```python
from build123d import *

# Parameters (mm, degrees)
SKETCH1_R                = 3.2639
BOSS_EXTRUDE1_DEPTH      = 6.35
SKETCH2_R                = 2.0193
CUT_EXTRUDE1_DEPTH       = 6.35
SKETCH3_R                = 2.0193
CUT_EXTRUDE2_DEPTH       = 6.35
SKETCH5_R                = 2.0193
CUT_EXTRUDE3_DEPTH       = 6.35
SKETCH6_R                = 14.2875
CUT_EXTRUDE4_DEPTH       = 7.35
SKETCH7_R                = 3.2639
CUT_EXTRUDE5_DEPTH       = 7.35
F_0_257_DIAMETER_HOLE1_D = 6.5278
FILLET1_R                = 3.175
FILLET2_R                = 3.175


with BuildPart() as part:
    # Sketch1 → Boss-Extrude1 (new body)
    with BuildSketch(Plane.XY):
        with BuildLine():
            Line((-12.7, 76.2), (12.7, 76.2))
            Line((12.7, 76.2), (12.7, -76.2))
            Line((12.7, -76.2), (3.175, -76.2))
            Line((3.175, -76.2), (-7.968733256, -102.786346034))
            ThreePointArc((-7.968733256, -102.786346034), (-15.132721636, -107.653920671), (-22.482997382, -103.072495258))
            Line((-22.482997382, -103.072495258), (-35.013847715, -76.2))
            Line((-35.013847715, -76.2), (-114.3, -76.2))
            Line((-114.3, -76.2), (-114.3, -25.4))
            Line((-114.3, -25.4), (-12.7, 76.2))
        make_face()
        with Locations((-15.289179323, -99.717962805)):
            Circle(SKETCH1_R, mode=Mode.SUBTRACT)
        with Locations((-20.656431247, -88.20785391)):
            Circle(SKETCH1_R, mode=Mode.SUBTRACT)
    extrude(amount=BOSS_EXTRUDE1_DEPTH)

    # Sketch2 → Cut-Extrude1 (cut)
    with BuildSketch(Plane.XY.offset(6.35)):
        with Locations((4.7625, 68.2625)):
            Circle(SKETCH2_R)
        with Locations((-4.7625, 58.7375)):
            Circle(SKETCH2_R)
    extrude(amount=-CUT_EXTRUDE1_DEPTH, mode=Mode.SUBTRACT)

    # Sketch3 → Cut-Extrude2 (cut)
    with BuildSketch(Plane.XY.offset(6.35)):
        with Locations((0, -63.5)):
            Circle(SKETCH3_R)
        with Locations((0, -38.1)):
            Circle(SKETCH3_R)
    extrude(amount=-CUT_EXTRUDE2_DEPTH, mode=Mode.SUBTRACT)

    # Sketch5 → Cut-Extrude3 (cut)
    with BuildSketch(Plane.XY.offset(6.35)):
        with Locations((-101.6, -63.5)):
            Circle(SKETCH5_R)
        with Locations((-101.6, -38.1)):
            Circle(SKETCH5_R)
    extrude(amount=-CUT_EXTRUDE3_DEPTH, mode=Mode.SUBTRACT)

    # Sketch6 → Cut-Extrude4 (cut, through all)
    with BuildSketch(Plane.XY.offset(6.35)):
        with Locations((-38.1, -50.8)):
            Circle(SKETCH6_R)
    extrude(amount=-CUT_EXTRUDE4_DEPTH, mode=Mode.SUBTRACT)

    # Sketch7 → Cut-Extrude5 (cut, through all)
    with BuildSketch(Plane.XY.offset(6.35)):
        with Locations((-57.15, -68.0339)):
            Circle(SKETCH7_R)
    extrude(amount=-CUT_EXTRUDE5_DEPTH, mode=Mode.SUBTRACT)

    # F (0.257) Diameter Hole1 (through all)
    with Locations(Plane.XY.offset(6.35)):
        with Locations((-82.55, -38.1), (-82.55, -63.5)):
            Hole(F_0_257_DIAMETER_HOLE1_D / 2)

    # Fillet1
    fillet1_edges = [part.edges().sort_by_distance(p)[0] for p in [
        (12.7, -76.2, 3.175),
        (3.175, -76.2, 3.175),
        (-35.013847715, -76.2, 3.175),
    ]]
    fillet(fillet1_edges, radius=FILLET1_R)

    # Fillet2
    fillet2_edges = [part.edges().sort_by_distance(p)[0] for p in [
        (-114.3, -76.2, 3.175),
        (-114.3, -25.4, 3.175),
        (-12.7, 76.2, 3.175),
        (12.7, 76.2, 3.175),
    ]]
    fillet(fillet2_edges, radius=FILLET2_R)


solid = part.part
```
Input: part model. Units: mm. Frame: model coordinates. A direction names the side the tool comes from. Coordinates: 2 decimals unless noted, no trailing zeros. Write each loop counter-clockwise with the first axis right and the second up, starting at its lowest first coordinate (ties: lowest second). Pieces come first, ordered by that corner, then holes. Notation, with made-up numbers: (33.25, 3) -> (87.25, 3) arc R31 cw to (87.25, 36) -> close; hole circle Ø6 at (20, -6.75). An arc over 180 degrees is marked (long way). Answer as a JSON object with one key per item and string values.
1. Mould query, pull axis Y, two halves, no side actions, for faces 3 (the face through (-36, -14, 6.35)), 4 (the face through (-23.06, -86, 3.13)), 5 (the face through (-103.09, -62.14, 3.22)), 6 (the face through (-28.24, -90.73, 3.13)). Classes: released by +Y, released by -Y, zero draft, split by the parting line, or undercut.
Result set:
{"face 3": "zero draft", "face 4": "undercut", "face 5": "undercut", "face 6": "released by -Y"}
2. Section A-A on x = -57.15. Return the cut outline in (y, z).
Result set:
{"outline": "(-76.2, 0) -> (-71.3, 0) -> (-71.3, 6.35) -> (-76.2, 6.35) -> close; (-64.77, 0) -> (31.75, 0) -> (31.75, 6.35) -> (-64.77, 6.35) -> close"}
3. Section D-D on z = 2. Count the separate pieces of the cut face and the enclosed holes in it, then the cut area to 3 significant figures.
Result set:
{"separate pieces": "1", "enclosed holes": "12", "area": "14,100 mm2"}
4. Material intervals for line 1 (Y direction, x = -82.55, z = 3); line 2 (X direction, y = -62, z = 2.75); line 3 (Y direction, x = -100, z = 0.75), sorted ascending. Write a range as from..to.
Result set:
{"line 1": "y = -76.2..-66.76, -60.24..-41.36, -34.84..6.35", "line 2": "x = -114.3..-102.95, -100.25..-85.45, -79.65..-46.97, -29.23..-1.35, 1.35..12.7", "line 3": "y = -76.2..-64.73, -62.27..-39.33, -36.87..-11.1"}
5. Section B-B on y = -50.8. Return the cut outline in (x, z).
Result set:
{"outline": "(-114.3, 0) -> (-52.39, 0) -> (-52.39, 6.35) -> (-114.3, 6.35) -> close; (-23.81, 0) -> (12.7, 0) -> (12.7, 6.35) -> (-23.81, 6.35) -> close"}
6. Access query for faces 1 (the face through (7, -76.2, 3)), 2 (the face through (1.09, -36.4, 3.22)). Directions: +Z, -Z, +X, -X, +Y, -Y. A direction counts if a zero-diameter tool reaches every point of the face in a straight line with its end or side. Return the directions, or none.
Result set:
{"face 1": "+Z, -Z, +X, -Y", "face 2": "+Z, -Z"}
7. Section C-C on x = 0. Return the cut outline in (y, z), then the cut area to 3 significant figures.
Result set:
{"outline": "(-83.77, 0) -> (-65.52, 0) -> (-65.52, 6.35) -> (-83.77, 6.35) -> close; (-61.48, 0) -> (-40.12, 0) -> (-40.12, 6.35) -> (-61.48, 6.35) -> close; (-36.08, 0) -> (76.2, 0) -> (76.2, 6.35) -> (-36.08, 6.35) -> close", "area": "965 mm2"}
8. First-contact query: P1, Ø2.5, axis at x = 0, y = -38.1, coming from the +Z side; P2, Ø4.5, axis at x = -4.76, y = 58.74, coming from the -Z side. Flat tips, straight axial feed; report the tip coordinate or a pass-through.
Result set:
{"P1": "passes through", "P2": "stops at z = 0"}
